Part model, mm, in its own coordinate system. A direction names the side the tool comes from. Round coordinates to 2 decimals unless told otherwise and drop trailing zeros. Write each loop counter-clockwise with the first axis right and the second up, starting at its lowest first coordinate (ties: lowest second). Pieces come first, ordered by that corner, then holes. Notation, with made-up numbers: M -8.5,64 L 43.5,64 A15 cw 43.5,90 Z; hole C 84,82 d7. An arc over 180 degrees is marked long. Answer as a JSON object with one key per item and string values. Group by question number.
1. Band-saw the part on B-B, the plane x = 34.5. Write the cut outline in (y, z).
2. Which spindle directions (+Z, -Z, +X, -X, +Y, -Y) get a long thin tool onto all of the face, cutting with end or side? Do faces 1 (the face through (-4, 85.072, 31)), 2 (the face through (-117.798, 24, 22)). Say none if no direction does.
3. Band-saw the part on A-A, the plane z = 53. Write the cut outline in (x, y).
4. Drill centre lines: line 1 (Y direction, x = -19, z = 18); line 2 (X direction, y = 31.5, z = 24); line 3 (X direction, y = -8, z = 3). Where is each one in solid material? Low to high. Write a range as from..to.
5. Two-plate mould, pull along Y, no slides. Class faces 3 (the face through (-5, 89.072, 29)), 4 (the face through (-5, -38.928, 29)), 5 (the face through (104, 85.072, 31)): +Y half, -Y half, draft (parallel to the pull), parting line (faces both ways), or undercut.
6. Band-saw the part on C-C, the plane x = 70.5. Write the cut outline in (y, z).
7. Drop a flat-ended pin along its axis: pin 1 (3 mm diameter, centred on x = 104.2, y = 82.07, fed in from +Z). Give the stop position or say it passes through.
from build123d import *

# Parameters (mm, degrees)
SKETCH_4_W                   = 229
SKETCH_4_H                   = 128
EXTRUDE_2_DEPTH              = 58
CUT_EXTRUDE_START            = 4
SKETCH_6_W                   = 221
SKETCH_6_H                   = 120
CUT_EXTRUDE_2_DEPTH          = 58
HOLE_WIZARD_M3_5_D           = 2.5
HOLE_WIZARD_M3_5_DEPTH       = 4
HOLE_WIZARD_M3_5_CSINK_D     = 3.05
HOLE_WIZARD_M3_5_CSINK_ANGLE = 90
HOLE_WIZARD_M3_3_D           = 2.5
HOLE_WIZARD_M3_3_CSINK_D     = 3.05
HOLE_WIZARD_M3_3_CSINK_ANGLE = 90
SKETCH_23_W                  = 5
SKETCH_23_H                  = 46
CUT_EXTRUDE_3_DEPTH          = 253.465633094
SKETCH_24_W                  = 41.070947304
SKETCH_24_H                  = 54
SKETCH_24_W_2                = 41
CUT_EXTRUDE_4_DEPTH          = 184.369425463
HOLE_WIZARD_M3_6_D           = 2.5
HOLE_WIZARD_M3_6_CSINK_D     = 3.05
HOLE_WIZARD_M3_6_CSINK_ANGLE = 90
HOLE_WIZARD_M3_7_D           = 2.5
HOLE_WIZARD_M3_7_CSINK_D     = 3.05
HOLE_WIZARD_M3_7_CSINK_ANGLE = 90
HOLE_WIZARD_M3_8_D           = 2.5
HOLE_WIZARD_M3_8_CSINK_D     = 3.05
HOLE_WIZARD_M3_8_CSINK_ANGLE = 90
HOLE_WIZARD_M3_9_D           = 2.5
HOLE_WIZARD_M3_9_CSINK_D     = 3.05
HOLE_WIZARD_M3_9_CSINK_ANGLE = 90
SKETCH_40_W                  = 5
SKETCH_40_H                  = 46
CUT_EXTRUDE_5_DEPTH          = 253.465633094
SKETCH_43_W                  = 12
SKETCH_43_H                  = 11.5
CUT_EXTRUDE_8_DEPTH          = 10.5


with BuildPart() as part:
    # 草图4 → 凸台-拉伸2 (new body)
    with BuildSketch(Plane.XY):
        with Locations((-3.297904033, 25.072419375)):
            Rectangle(SKETCH_4_W, SKETCH_4_H)
    extrude(amount=EXTRUDE_2_DEPTH)

    # 草图6 → 切除-拉伸2 (cut)
    with BuildSketch(Plane.XY.offset(CUT_EXTRUDE_START)):
        with Locations((-3.297904033, 25.072419375)):
            Rectangle(SKETCH_6_W, SKETCH_6_H)
    extrude(amount=CUT_EXTRUDE_2_DEPTH, mode=Mode.SUBTRACT)

    # M3 螺纹孔5
    with Locations(Plane(origin=(111.202095967, 0, 0), x_dir=(0, 0, -1), z_dir=(1, 0, 0))):
        with Locations((-46, 69.072419375), (-12, 69.072419375), (-12, -18.927580625), (-46, -18.927580625)):
            CounterSinkHole(HOLE_WIZARD_M3_5_D / 2, HOLE_WIZARD_M3_5_CSINK_D / 2, depth=HOLE_WIZARD_M3_5_DEPTH, counter_sink_angle=HOLE_WIZARD_M3_5_CSINK_ANGLE)

    # M3 螺纹孔3 (through all)
    with Locations(Plane(origin=(-117.797904033, 69.072419375, 12), x_dir=(0, 0, -1), z_dir=(-1, 0, 0))):
        with Locations((0, 0), (-34, 0), (-34, 88), (0, 88)):
            CounterSinkHole(HOLE_WIZARD_M3_3_D / 2, HOLE_WIZARD_M3_3_CSINK_D / 2, counter_sink_angle=HOLE_WIZARD_M3_3_CSINK_ANGLE)

    # 草图23 → 切除-拉伸3 (cut, through all)
    with BuildSketch(Plane.ZY.offset(117.797904033)):
        with Locations((47.5, 25.072419375)):
            Rectangle(SKETCH_23_W, SKETCH_23_H)
    extrude(amount=-CUT_EXTRUDE_3_DEPTH, mode=Mode.SUBTRACT)

    # 草图24 → 切除-拉伸4 (cut, through all)
    with BuildSketch(Plane.XZ.offset(38.927580625)):
        with Locations((-87.333377685, 31)):
            Rectangle(SKETCH_24_W, SKETCH_24_H)
        with Locations((80.702095967, 31)):
            Rectangle(SKETCH_24_W_2, SKETCH_24_H)
    extrude(amount=-CUT_EXTRUDE_4_DEPTH, mode=Mode.SUBTRACT)

    # M3 螺纹孔6 (through all)
    with Locations(Plane(origin=(0, 0, 0), x_dir=(-1, 0, 0), z_dir=(0, 0, -1))):
        with Locations((-104.202095967, 82.072419375), (-104.202095967, -31.927580625), (110.797904033, -31.927580625), (110.797904033, 82.072419375)):
            CounterSinkHole(HOLE_WIZARD_M3_6_D / 2, HOLE_WIZARD_M3_6_CSINK_D / 2, counter_sink_angle=HOLE_WIZARD_M3_6_CSINK_ANGLE)

    # M3 螺纹孔7 (through all)
    with Locations(Plane.XY.offset(4)):
        with Locations((-5.997904033, -18.927580625), (-11.077904033, 31.872419375), (-39.017904033, 31.872419375), (-54.257904033, -18.927580625)):
            CounterSinkHole(HOLE_WIZARD_M3_7_D / 2, HOLE_WIZARD_M3_7_CSINK_D / 2, counter_sink_angle=HOLE_WIZARD_M3_7_CSINK_ANGLE)

    # M3 螺纹孔8 (through all)
    with Locations(Plane.XY.offset(4)):
        with Locations((10.202095967, 44.072419375), (10.202095967, 81.072419375), (47.202095967, 81.072419375), (47.202095967, 44.072419375), (47.202095967, 6.072419375), (47.202095967, -30.927580625), (10.202095967, -30.927580625), (10.202095967, 6.072419375)):
            CounterSinkHole(HOLE_WIZARD_M3_8_D / 2, HOLE_WIZARD_M3_8_CSINK_D / 2, counter_sink_angle=HOLE_WIZARD_M3_8_CSINK_ANGLE)

    # M3 螺纹孔9 (through all)
    with Locations(Plane.XY.offset(4)):
        with Locations((-102.260717179, 80.197574321), (-102.059054013, 55.998414584), (-72.060095662, 56.248410244), (-72.261758827, 80.44756998), (65.702095967, 81.022419375), (95.702095967, 81.022419375), (95.702095967, 56.822419375), (65.702095967, 56.822419375), (65.702095967, -6.677580625), (95.702095967, -6.677580625), (95.702095967, -30.877580625), (65.702095967, -30.877580625), (-71.329275016, -31.44854467), (-71.530938182, -7.249384934), (-101.529896533, -7.499380593), (-101.328233368, -31.69854033)):
            CounterSinkHole(HOLE_WIZARD_M3_9_D / 2, HOLE_WIZARD_M3_9_CSINK_D / 2, counter_sink_angle=HOLE_WIZARD_M3_9_CSINK_ANGLE)

    # 草图40 → 切除-拉伸5 (cut, through all)
    with BuildSketch(Plane.ZY.offset(117.797904033)):
        with Locations((28.5, 25.072419375)):
            Rectangle(SKETCH_40_W, SKETCH_40_H)
    extrude(amount=-CUT_EXTRUDE_5_DEPTH, mode=Mode.SUBTRACT)

    # 草图43 → 切除-拉伸8 (cut)
    with BuildSketch(Plane.XZ.offset(38.927580625)):
        with Locations((-40.797904033, 11)):
            Rectangle(SKETCH_43_W, SKETCH_43_H)
    extrude(amount=-CUT_EXTRUDE_8_DEPTH, mode=Mode.SUBTRACT)


solid = part.part
Worked answers:
{
 "1": {"outline": "M -38.93,0 L 89.07,0 L 89.07,58 L 85.07,58 L 85.07,4 L -34.93,4 L -34.93,58 L -38.93,58 Z"},
 "2": {"face 1": "+Z", "face 2": "+Z, -Z, -X, +Y, -Y"},
 "3": {"outline": "M -117.8,-38.93 L -107.87,-38.93 L -107.87,-34.93 L -113.8,-34.93 L -113.8,85.07 L -107.87,85.07 L -107.87,89.07 L -117.8,89.07 Z; M -66.8,-38.93 L 60.2,-38.93 L 60.2,-34.93 L -66.8,-34.93 Z; M -66.8,85.07 L 60.2,85.07 L 60.2,89.07 L -66.8,89.07 Z; M 101.2,-38.93 L 111.2,-38.93 L 111.2,89.07 L 101.2,89.07 L 101.2,85.07 L 107.2,85.07 L 107.2,-34.93 L 101.2,-34.93 Z"},
 "4": {"line 1": "y = -38.93..-34.93, 85.07..89.07", "line 2": "x = -117.8..-113.8, 107.2..111.2", "line 3": "x = -117.8..-102.68, -100.38..-72.53, -70.53..111.2"},
 "5": {"face 3": "+Y half", "face 4": "-Y half", "face 5": "undercut"},
 "6": {"outline": "M -38.93,0 L 89.07,0 L 89.07,4 L -38.93,4 Z"},
 "7": {"pin 1": "stops at z = 4"}
}
